Part print with two shaded views. Sizes in mm from the minimum x, y, z corner. A direction names the side the tool comes from. Round coordinates to 2 decimals unless told otherwise and drop trailing zeros. Write each loop counter-clockwise with the first axis right and the second up, starting at its lowest first coordinate (ties: lowest second). Pieces come first, ordered by that corner, then holes. Notation, with made-up numbers: (-3.5, 6) -> (53.5, 6) arc R14 ccw to (53.5, 31) -> close; hole circle Ø9 at (65.5, -36.75). An arc over 180 degrees is marked (long way). Return JSON: item names as keys, results as strings. Group by question number.
(1) Saw through at A-A (x = 5.08). List the corners of the cut face in (y, z), plus the area to 3 significant figures.
(2) Saw through at B-B (z = 41.5). List the corners of the cut face in (x, y).
(3) Saw through at D-D (z = 28.5). List the corners of the cut face in (x, y).
(4) Drop flat-ended pins along their axis: pin 1 Ø6 at (x, z) = (6, 30.5) entering from +Y; pin 2 Ø5 at (x, y) = (24.892, 70.866) entering from +Z; pin 3 Ø10 at (x, z) = (25.5, 11.5) entering from +Y. Give the stop position or say it passes through.
(5) Tool access for the marked faces 4, 5 and 6: list every direction of +Z, -Z, +X, -X, +Y, -Y with a clear straight run to the whole face (end or side of a thin tool).
(6) Drill centre lines: L1, parallel to Y at x = 5.08, z = 1.75; L2, parallel to Z at x = 23.75, y = 59.5; L3, parallel to Y at x = 29, z = 16.5. Where is each one in solid material? Low to high. Write a range as from..to.
(7) Saw through at C-C (y = 11.5). List the corners of the cut face in (x, z), plus the area to 3 significant figures.
(8) Mould opens along X. For the marked faces 1, 2 and 3 say: +X half, -X half, draft (parallel to the pull), parting line (faces both ways), or undercut.
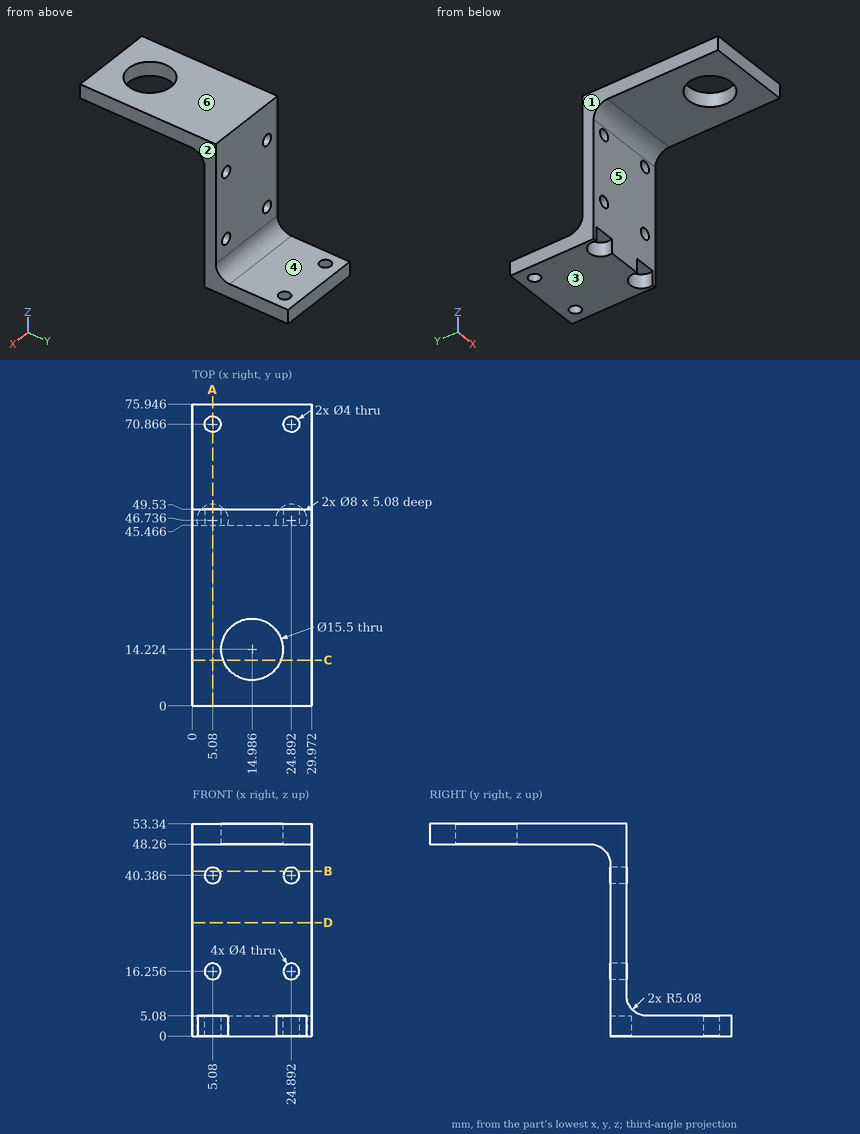
Computed values:
{
 "1": {"outline": "(0, 48.26) -> (40.39, 48.26) arc R5.08 cw to (45.47, 43.18) -> (45.47, 42.39) -> (49.53, 42.39) -> (49.53, 53.34) -> (0, 53.34) -> close; (45.47, 5.08) -> (50.74, 5.08) -> (50.74, 0) -> (68.87, 0) -> (68.87, 5.08) -> (54.61, 5.08) arc R5.08 cw to (49.53, 10.16) -> (49.53, 14.26) -> (45.47, 14.26) -> close; (45.47, 18.26) -> (49.53, 18.26) -> (49.53, 38.39) -> (45.47, 38.39) -> close; (72.87, 0) -> (75.95, 0) -> (75.95, 5.08) -> (72.87, 5.08) -> close", "area": "513 mm2"},
 "2": {"outline": "(0, 45.47) -> (3.42, 45.47) -> (3.42, 49.53) -> (0, 49.53) -> close; (6.74, 45.47) -> (23.23, 45.47) -> (23.23, 49.53) -> (6.74, 49.53) -> close; (26.55, 45.47) -> (29.97, 45.47) -> (29.97, 49.53) -> (26.55, 49.53) -> close"},
 "3": {"outline": "(0, 45.47) -> (29.97, 45.47) -> (29.97, 49.53) -> (0, 49.53) -> close"},
 "4": {"pin 1": "y = 49.53", "pin 2": "z = 5.08", "pin 3": "y = 51.09"},
 "5": {"face 4": "+Z, +X, -X, +Y", "face 5": "-Z, +X, -X, -Y", "face 6": "+Z, +X, -X, +Y, -Y"},
 "6": {"L1": "50.74..68.87, 72.87..75.95", "L2": "0..5.08", "L3": "45.47..49.53"},
 "7": {"outline": "(0, 48.26) -> (7.73, 48.26) -> (7.73, 53.34) -> (0, 53.34) -> close; (22.24, 48.26) -> (29.97, 48.26) -> (29.97, 53.34) -> (22.24, 53.34) -> close", "area": "78.5 mm2"},
 "8": {"face 1": "-X half", "face 2": "+X half", "face 3": "draft"}
}
